Design review of the part built by this model. Coordinates are the model's own, in mm. A direction names the side the tool comes from. Give positions to 0.01 mm unless a question says otherwise; leave off trailing zeros. Order: outer loops, then holes, each group sorted by start corner. A loop starts at its lowest first (then second) coordinate and runs counter-clockwise, first axis right, second up. Notation, with made-up numbers: (64.5, -11) -> (76.5, -11) arc R35 ccw to (76.5, 25) -> close; hole circle Ø2 at (-6, 34.5). An arc over 180 degrees is marked (long way). Return JSON: item names as keys, results as strings.
Autodesk Inventor part; units mm, degrees
ref_plane "Work Plane1" through (44.45, 0, 0) normal (1, 0, 0) x (0, 1, 0)
ref_plane "XZ Plane" through (0, 0, 0) normal (0, 1, 0) x (-1, 0, 0)
ref_plane "XY Plane" through (0, 0, 0) normal (0, 0, 1) x (1, 0, 0)
sketch "Sketch1" plane through (0, 0, 0) normal (0, 0, 1) x (1, 0, 0)
  circle A0 centre (0, 0) radius 44.45
  line L0 (-32.2263, -21.7487) -> (32.2263, -21.7487) construction
  line L1 (32.2263, -21.7487) -> (32.2263, 21.7487)
  line L2 (32.2263, 21.7487) -> (-32.2263, 21.7487) construction
  line L3 (-32.2263, 21.7487) -> (-32.2263, -21.7487) construction
  line L4 (-32.2263, -21.7487) -> (32.2263, 21.7487) construction
  line L5 (32.2263, -21.7487) -> (-32.2263, 21.7487) construction
  line L6 (-23.8125, -30.1625) -> (23.8125, -30.1625) construction
  line L7 (23.8125, -30.1625) -> (23.8125, 30.1625) construction
  line L8 (23.8125, 30.1625) -> (-23.8125, 30.1625) construction
  line L9 (-23.8125, 30.1625) -> (-23.8125, -30.1625) construction
  line L10 (-23.8125, -30.1625) -> (23.8125, 30.1625) construction
  line L11 (23.8125, -30.1625) -> (-23.8125, 30.1625) construction
  line L12 (-32.2263, 21.7487) -> (-23.8125, 30.1625) construction
  line L13 (-32.2263, -21.7487) -> (-23.8125, -30.1625) construction
  line L14 (23.8125, -30.1625) -> (32.2263, -21.7487) construction
  line L15 (32.2263, 21.7487) -> (23.8125, 30.1625) construction
  line L16 (32.2263, 0) -> (44.45, 0) construction
  line L17 (40.1609, 19.05) -> (32.2263, 19.05)
  line L18 (32.2263, -19.05) -> (40.1609, -19.05)
  dimension "d0" = 88.9
  dimension "d2" = 64.4525
  dimension "d5" = 47.625
  dimension "d6" = 60.325
  dimension "d18" = 45
  dimension "d22" = 19.05
  dimension "d23" = 19.05
extrude "Extrusion1" add sketch "Sketch1" along normal blind 9.525 contours A0 L18 L1 L17 picked at (36.3009, 0)
ref_plane "Work Plane1" through (44.45, 0, 0) normal (1, 0, 0) x (0, 1, 0)
sketch "Sketch2" plane through (44.45, 0, 0) normal (1, 0, 0) x (0, 1, 0)
  line L0 (0, 9.9848) -> (0, 0) construction
  line L1 (-19.05, 4.7625) -> (19.05, 4.7625) construction
  line L2 (19.05, 0) -> (-19.05, 0)
  line L3 (-19.05, 0) -> (-19.05, 9.525)
  line L4 (19.05, 9.525) -> (-19.05, 9.525)
  line L5 (19.05, 0) -> (19.05, 9.525)
  point P0 (-9.525, 4.7625)
  point P1 (9.525, 4.7625)
  dimension "d9" = 19.05
  dimension "d10" = 9.525
hole "Hole2" at (44.45, -9.525, 4.7625) at (44.45, 9.525, 4.7625) direction (-1, 0, 0) diameter 3.6576 end through all counterbore diameter 6.858 counterbore depth 4.445
properties part number "Radial Bushing"
Item 1: For pin 1 (6 mm diameter, centred on x = 42, y = 0.5, fed in from -Z); pin 2 (5.5 mm diameter, centred on y = -10.5, z = 5, fed in from +X), all flat-tipped, find the tip position at first contact; note any pin that passes through.
Result set:
{"pin 1": "stops at z = 0", "pin 2": "stops at x = 42.93"}
Item 2: Mouldability with a two-part tool opening along Y and no side actions: class faces 3 (the face through (32.226, 0, 5)), 4 (the face through (36, -19.05, 5)), 5 (the face through (36.06, -7.74, 5.16)) as released by +Y, released by -Y, zero draft, split by the parting line, or undercut.
Result set:
{"face 3": "zero draft", "face 4": "released by -Y", "face 5": "undercut"}
Item 3: Wall thickness on L1, parallel to Y at x = 35.5, z = 5.75; L2, parallel to X at y = -8, z = 2.25 (3 decimals); L3, parallel to X at y = 0.5, z = 2.75: over which ranges is each line inside the solid? List them lowest first. Write a range as [from, to].
Result set:
{"L1": "y = [-19.05, -11.06], [-7.99, 7.99], [11.06, 19.05]", "L2": "x = [32.226, 40.005]", "L3": "x = [32.23, 44.45]"}
Item 4: Add section A-A (z = 5.75). Give the boundary of the cut face in (x, y) (3 decimals).
Result set:
{"outline": "(32.226, -19.05) -> (40.161, -19.05) arc R44.45 ccw to (42.565, -12.809) -> (40.005, -12.809) -> (40.005, -11.064) -> (32.226, -11.064) -> close; (32.226, -7.986) -> (40.005, -7.986) -> (40.005, -6.241) -> (44.01, -6.241) arc R44.45 ccw to (44.01, 6.241) -> (40.005, 6.241) -> (40.005, 7.986) -> (32.226, 7.986) -> close; (32.226, 11.064) -> (40.005, 11.064) -> (40.005, 12.809) -> (42.565, 12.809) arc R44.45 ccw to (40.161, 19.05) -> (32.226, 19.05) -> close"}
Item 5: Machinability: for faces 1 (the face through (38, 0, 9.525)), 2 (the face through (41.54, -6.18, 5.51)), which of the approach directions +Z, -Z, +X, -X, +Y, -Y give a long, thin tool a straight path to every point of the face, cutting with its end or side? Answer none if there is none.
Result set:
{"face 1": "+Z, +X, -X, +Y, -Y", "face 2": "+X"}
Item 6: Add section B-B (x = 41). Give the boundary of the cut face in (y, z) (1 decimal).
Result set:
{"outline": "(-17.2, 0) -> (17.2, 0) -> (17.2, 9.5) -> (-17.2, 9.5) -> close; hole circle Ø6.9 at (-9.5, 4.8); hole circle Ø6.9 at (9.5, 4.8)"}
Item 7: Add section C-C (y = 10.5). Give the boundary of the cut face in (x, z) (3 decimals), plus the area to 3 significant figures.
Result set:
{"outline": "(32.226, 0) -> (43.192, 0) -> (43.192, 1.475) -> (40.005, 1.475) -> (40.005, 3.215) -> (32.226, 3.215) -> close; (32.226, 6.31) -> (40.005, 6.31) -> (40.005, 8.05) -> (43.192, 8.05) -> (43.192, 9.525) -> (32.226, 9.525) -> close", "area": "59.4 mm^2"}
Item 8: Add section D-D (y = -12). Give the boundary of the cut face in (x, z) (3 decimals).
Result set:
{"outline": "(32.226, 0) -> (42.8, 0) -> (42.8, 2.389) -> (40.005, 2.389) -> (40.005, 7.136) -> (42.8, 7.136) -> (42.8, 9.525) -> (32.226, 9.525) -> close"}
